CAD build for the part. Positions are in the model's coordinates, mm. Face numbers are marked on the shaded views. Round coordinates to 2 decimals unless told otherwise and drop trailing zeros. Order: outer loops, then holes, each group sorted by start corner. A loop starts at its lowest first (then second) coordinate and runs counter-clockwise, first axis right, second up.
```python
from build123d import *

# Parameters (mm, degrees)
F0_R      = 33.15
F1_DEPTH  = 57.5
F3_DEPTH  = 5
F8_DEPTH  = 5
F9_DEPTH  = 3.048
F10_R     = 28.5244197483
F11_DEPTH = 6.35
F14_DEPTH = 1.5


# Not quite as in the source:
# - a feature names something its author has since deleted; it is built from what else it names


with BuildPart() as f1:
    # F0 (on Top) → F1 (new body, symmetric)
    with BuildSketch(Plane.XY):
        Circle(F0_R)
    extrude(amount=F1_DEPTH, both=True)

    # F2 (on face) → F3 (join)
    with BuildSketch(Plane.XY.offset(57.5)):
        with BuildLine():
            ThreePointArc((27.5449306971, 7.4107567004), (-28.2784872926, -3.7376032987), (28.5244197483, 0))
            ThreePointArc((28.5244197483, 0), (28.2784872926, 3.7376032987), (27.5449306971, 7.4107567004))
        make_face()
        with BuildLine():
            Line((-3.6688328255, 16.6036896408), (0, 16.6036896408))
            Line((0, 16.6036896408), (3.6688328255, 16.6036896408))
            ThreePointArc((3.6688328255, 16.6036896408), (4.3933325809, 16.3940702991), (4.8939753324, 15.8299807676))
            Line((4.8939753324, 15.8299807676), (4.6938681044, 5.1092766225))
            ThreePointArc((4.6938681044, 5.1092766225), (3.3149072999, 1.6653658978), (0, 0))
            ThreePointArc((0, 0), (-3.3149072999, 1.6653658978), (-4.6938681044, 5.1092766225))
            Line((-4.6938681044, 5.1092766225), (-4.8939753324, 15.8299807676))
            ThreePointArc((-4.8939753324, 15.8299807676), (-4.3933325809, 16.3940702991), (-3.6688328255, 16.6036896408))
        make_face(mode=Mode.SUBTRACT)
    extrude(amount=F3_DEPTH)

    # F7: F6 across plane


with BuildPart() as f6:
    # F4 (on Front) → F6 (revolve)
    with BuildSketch(Plane.XZ):
        with BuildLine():
            add(Edge.make_bspline(
                [(28.5244197483, 62.5), (28.9434660226, 59.606384486), (31.2671773136, 57.7946938574), (33.15, 57.5)],
                knots=[0, 0, 0, 0, 6.8114603915, 6.8114603915, 6.8114603915, 6.8114603915], degree=3))
            Line((28.5244197483, 62.5), (28.5244197483, 57.5))
            Line((28.5244197483, 57.5), (33.15, 57.5))
        make_face()
    revolve(axis=Axis((0, 0, 67.1579949558), (0, 0, 1)))


with BuildPart() as f1_1:
    add(f1.part)
    add(f6.part.mirror(Plane.XY))

    # F8 (add): a face of the model
    f8_faces = [f1_1.faces().sort_by_distance(p)[0] for p in [
        (0, 0, -57.5),
    ]]
    extrude(f8_faces, amount=F8_DEPTH)

    # F9 (add): a face of the model
    f9_faces = [f1_1.faces().sort_by_distance(p)[0] for p in [
        (0, -0.5407612008, 62.5),
    ]]

    add(f6.part)  # F9 merges F6
    extrude(f9_faces, amount=-F9_DEPTH)

    # F10 (on face) → F11 (cut)
    with BuildSketch(Plane.XY.offset(62.5)):
        Circle(F10_R)
    extrude(amount=-F11_DEPTH, mode=Mode.SUBTRACT)

    # F13 (on face) → F14 (join)
    with BuildSketch(Plane.XY.offset(56.15)):
        with BuildLine():
            Line((3.6663445585, 18.275173819), (-0.002488267, 18.275173819))
            Line((-0.002488267, 18.275173819), (-3.6713210925, 18.275173819))
            ThreePointArc((-3.6713210925, 18.275173819), (-4.395820848, 18.0655544773), (-4.8964635994, 17.5014649459))
            Line((-4.8964635994, 17.5014649459), (-4.6963563714, 6.7807608008))
            ThreePointArc((-4.6963563714, 6.7807608008), (-3.3173955669, 3.336850076), (-0.002488267, 1.6714841783))
            ThreePointArc((-0.002488267, 1.6714841783), (3.3124190329, 3.336850076), (4.6913798374, 6.7807608008))
            Line((4.6913798374, 6.7807608008), (4.8914870654, 17.5014649459))
            ThreePointArc((4.8914870654, 17.5014649459), (4.3908443139, 18.0655544773), (3.6663445585, 18.275173819))
        make_face()
        with BuildLine():
            ThreePointArc((-0.002488267, 8.3136439422), (1.6104378587, 6.7007178165), (-0.002488267, 5.0877916907))
            ThreePointArc((-0.002488267, 5.0877916907), (-1.6154143928, 6.7007178165), (-0.002488267, 8.3136439422))
        make_face(mode=Mode.SUBTRACT)
        with BuildLine():
            ThreePointArc((-0.002488267, 17.4195373118), (3.997511733, 13.4195373118), (-0.002488267, 9.4195373118))
            ThreePointArc((-0.002488267, 9.4195373118), (-4.002488267, 13.4195373118), (-0.002488267, 17.4195373118))
        make_face(mode=Mode.SUBTRACT)
    extrude(amount=F14_DEPTH)


solid = f1_1.part
```
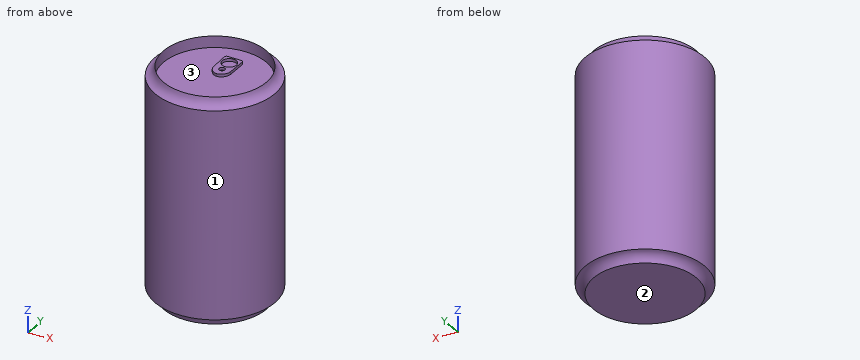
1. Pin check, flat tips, straight feed: P1, Ø1.6, axis at x = -0.5, z = 57, coming from the +Y side; P2, Ø1, axis at x = 18, y = 20.5, coming from the +Z side; P3, Ø5, axis at x = -26, z = 6, coming from the -Y side. Stop position of each tip, or through.
2. Mould opens along X. For the marked faces 1, 2 and 3 say: released by +X, released by -X, zero draft, split by the parting line, or undercut.
3. Drill centre lines: line 1 (Z direction, x = 3.5, y = -13); line 2 (Y direction, x = 0, z = 61); line 3 (X direction, y = 0, z = 58). Where is each one in solid material? Low to high.
4. Cut at A-A, the plane z = 52.5. Write the cut outline in (x, y).
Outcome:
1. P1: stops at y = 33.15
1. P2: stops at z = 56.15
1. P3: stops at y = -23.38
2. face 1: split by the parting line
2. face 2: zero draft
2. face 3: undercut
3. line 1: z = -62.5 to 56.15
3. line 2: y = -28.94 to -28.52, 28.52 to 28.94
3. line 3: x = -31.69 to -28.52, 28.52 to 31.69
4. outline: circle Ø66.3 at (0, 0)
